from build123d import *

# Parameters (mm, degrees)
SKETCH1_W           = 24
SKETCH1_H           = 24
BOSS_EXTRUDE1_DEPTH = 8
SKETCH2_OUTSIDE_W   = 60.688
SKETCH2_OUTSIDE_H   = 60.688
SKETCH2_OUTSIDE_R   = 11.874068454
CUT_EXTRUDE1_DEPTH  = 8
CUT_EXTRUDE1_DRAFT  = -60
SKETCH3_R           = 6
BOSS_EXTRUDE2_DEPTH = 98
CHAMFER1_SIZE       = 1


with BuildPart() as part:
    # Sketch1 → Boss-Extrude1 (new body)
    with BuildSketch(Plane(origin=(0, 0, 0), x_dir=(1, 0, 0), z_dir=(0, 1, 0))):
        Rectangle(SKETCH1_W, SKETCH1_H)
    extrude(amount=BOSS_EXTRUDE1_DEPTH)


with BuildPart() as cut_extrude1_tool:
    # Sketch2 outside → Cut-Extrude1 (with draft: the straight prism first)
    with BuildSketch(Plane(origin=(0, 8, 0), x_dir=(1, 0, 0), z_dir=(0, 1, 0))):
        Rectangle(SKETCH2_OUTSIDE_W, SKETCH2_OUTSIDE_H)
        Circle(SKETCH2_OUTSIDE_R, mode=Mode.SUBTRACT)
    extrude(amount=-CUT_EXTRUDE1_DEPTH)
    # Cut-Extrude1: the draft: its side faces are tilted about the plane it starts from
    cut_extrude1_sides = [cut_extrude1_tool.faces().sort_by_distance(p)[0] for p in [
        (0, 4, 30.344),
        (30.344, 4, 0),
        (0, 4, -30.344),
        (-30.344, 4, 0),
        (-11.874068454, 4, 0),
    ]]
    draft(cut_extrude1_sides, Plane(origin=(0, 8, 0), x_dir=(1, 0, 0), z_dir=(0, 1, 0)), CUT_EXTRUDE1_DRAFT)


with BuildPart() as part_1:
    add(part.part)

    # Cut-Extrude1: cut by cut_extrude1_tool
    add(cut_extrude1_tool.part, mode=Mode.SUBTRACT)

    # Sketch3 → Boss-Extrude2 (add)
    with BuildSketch(Plane.XZ):
        with Locations(Location((0, 0, 0), (0, 0, 270))):
            Circle(SKETCH3_R)
    extrude(amount=BOSS_EXTRUDE2_DEPTH)

    # Chamfer1
    chamfer1_edges = [part_1.edges().sort_by_distance(p)[0] for p in [
        (0, -98, 6),
    ]]
    chamfer(chamfer1_edges, length=CHAMFER1_SIZE)


solid = part_1.part
The listing builds one solid part. Answer for the finished solid, in the listing's coordinates (mm). A direction names the side the tool comes from. Give positions to 0.01 mm unless a question says otherwise; leave off trailing zeros. Loops run counter-clockwise (first coordinate to the right, second up) from the corner with the lowest first, then second, coordinate; pieces in that order, holes last. Notation, with made-up numbers: M 82,35 L 123,35 A14 ccw 123,46 Z; hole C 3,-34.75 d1. An arc over 180 degrees is marked long. Answer as CSV lines item,"result".
Item 1: Straight lines are drawn through the part: line 1 along Y through (x, z) = (-3, -7.25); line 2 along Z through (x, y) = (-0.5, -54); line 3 along Y through (x, z) = (5, -0.25). For each, find the intervals that lie inside material, in ascending order. Write a range as [from, to].
Values follow:
line 1,"y = [0, 8]"
line 2,"z = [-5.98, 5.98]"
line 3,"y = [-97.99, 8]"
Item 2: Which of the six approach directions +Z, -Z, +X, -X, +Y, -Y give full straight-line access (tool end or side, diameter ignored) to faces 1 (the cylindrical face through (1.802, -47.821, -5.723)), 2 (the flat face through (0, 3, -12))?
Values follow:
face 1,"-Y"
face 2,"-Z, +X, -X, +Y, -Y"
Item 3: The part is cut by section B-B (x = 0). Give the vertices of the cut face in (y, z).
Values follow:
outline,"M -98,-5 L -97,-6 L 0,-6 L 0,-12 L 7.93,-12 L 8,-11.87 L 8,11.87 L 7.93,12 L 0,12 L 0,6 L -97,6 L -98,5 Z"
Item 4: The part is cut by section A-A (z = 0). Give the vertices of the cut face in (x, y), and give its area (3 significant figures).
Values follow:
outline,"M -12,0 L -6,0 L -6,-97 L -5,-98 L 5,-98 L 6,-97 L 6,0 L 12,0 L 12,7.93 L 11.87,8 L -11.87,8 L -12,7.93 Z"
area,"1,370 mm^2"
Item 5: Given pin 1 Ø1 at (y, z) = (-3, 4) entering from -X; pin 2 Ø1.5 at (x, z) = (-7, 8.5) entering from -Y; pin 3 Ø3 at (y, z) = (-44, 1.5) entering from +X; pin 4 Ø10 at (x, z) = (-6, -5) entering from -Y, each flat-ended and moving along its own axis, determine where each tip first touches the part or whether it passes through.
Values follow:
pin 1,"stops at x = -4.87"
pin 2,"stops at y = 0"
pin 3,"stops at x = 6"
pin 4,"stops at y = -98"
Item 6: The part is cut by section C-C (y = -1). Give the vertices of the cut face in (x, z), and give its area (3 significant figures).
Values follow:
outline,"C 0,0 d12"
area,"113 mm^2"
